Can you work these out from the model? Positions are in its coordinate system, mm. Face numbers are marked on the shaded views. Coordinates: 2 decimals unless noted, no trailing zeros. Loops run counter-clockwise (first coordinate to the right, second up) from the corner with the lowest first, then second, coordinate; pieces in that order, holes last. Notation, with made-up numbers: (-5.75, 26) -> (53.25, 26) arc R26 cw to (53.25, 47) -> close; hole circle Ø3 at (69.5, -1). An arc over 180 degrees is marked (long way). Put each result on its own line as item: value. Start each with the question number.
Item 1: If we section it at A-A on x = -34.75: Please give me the cut outline in (y, z).
Item 2: Will this pin go through, and if not, where does the flat tip stop? P1, Ø5, axis at y = -12.5, z = -5.5, coming from the -X side.
Item 3: If we section it at D-D on z = -4.5: Please give me the cut outline in (x, y), plus the area to 3 significant figures.
Item 4: If we section it at B-B on y = -17.5: Please give me the cut outline in (x, z), plus the area to 3 significant figures.
Item 5: We'd pull the mould along X, two halves only. Please class the marked faces 1, 2 and 3: pulls with the +X half, pulls with the -X half, needs draft (parallel to the pull), parting line crosses it, or undercut.
Item 6: Please list where these lines run through material, in increasing order: L1, parallel to X at y = -5.75, z = 0; L2, parallel to Z at x = -32, y = -3.75; L3, parallel to Z at x = -38, y = -3. Write a range as from..to.
Item 7: If we section it at C-C on z = 0: Please give me the cut outline in (x, y), plus the area to 3 significant figures.
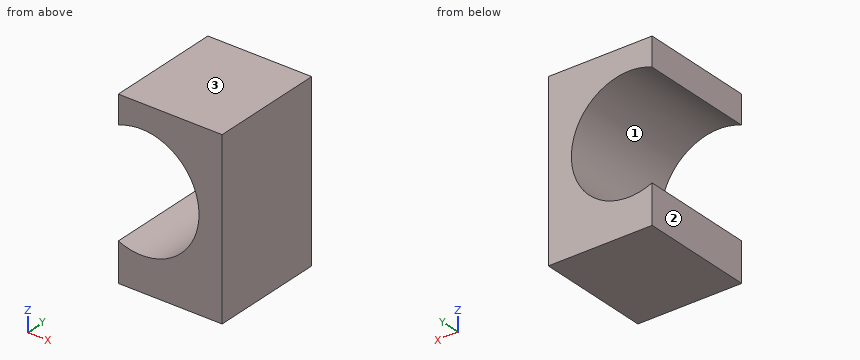
```python
from build123d import *

# Parameters (mm, degrees)
F0_W     = 22.86
F0_H     = 38.1
F1_DEPTH = 25.4
F2_R     = 12.7
F3_DEPTH = 89
F5_DEPTH = 25.401


# Not quite as in the source:
# - an extrude ends at something that could not be found from the text; its depth is read off the source's solid


with BuildPart() as f1:
    # F0 (on Front) → F1 (new body)
    with BuildSketch(Plane.XZ):
        with Locations((-34.8423583888, -1.1378988595)):
            Rectangle(F0_W, F0_H)
    extrude(amount=F1_DEPTH)

    # F2 (on Front) → F3 (cut, through all)
    with BuildSketch(Plane.XZ):
        with Locations((-35.3627614677, 3.7935657892)):
            Circle(F2_R)
    extrude(amount=-F3_DEPTH, mode=Mode.SUBTRACT)

    # F4 (on face) → F5 (cut, through all)
    with BuildSketch(Plane(origin=(0, 0, 0), x_dir=(-1, 0, 0), z_dir=(0, 1, 0))):
        with BuildLine():
            ThreePointArc((46.2723583888, -11.6417417865), (51.8211548639, -6.9581684388), (53.8969423294, 0))
            ThreePointArc((53.8969423294, 0), (51.8211548639, 6.9581684388), (46.2723583888, 11.6417417865))
            Line((46.2723583888, 11.6417417865), (46.2723583888, -11.6417417865))
        make_face()
        with BuildLine():
            Line((46.2723583888, -11.6417417865), (46.2723583888, 11.6417417865))
            ThreePointArc((46.2723583888, 11.6417417865), (28.4969423294, 0), (46.2723583888, -11.6417417865))
        make_face()
    extrude(amount=-F5_DEPTH, mode=Mode.SUBTRACT)


solid = f1.part
```
Solutions:
1. outline: (-25.4, -20.19) -> (0, -20.19) -> (0, -10.94) -> (-25.4, -10.94) -> close; (-25.4, 10.94) -> (0, 10.94) -> (0, 17.91) -> (-25.4, 17.91) -> close
2. P1: x = -31.33
3. outline: (-29.32, -25.4) -> (-23.41, -25.4) -> (-23.41, 0) -> (-29.32, 0) -> close
3. area: 150 mm^2
4. outline: (-46.27, -20.19) -> (-23.41, -20.19) -> (-23.41, 17.91) -> (-46.27, 17.91) -> (-46.27, 11.64) arc R12.7 cw (long way) to (-46.27, -11.64) -> close
4. area: 492 mm^2
5. face 1: undercut
5. face 2: pulls with the -X half
5. face 3: needs draft
6. L1: -28.5..-23.41
6. L2: -20.19..-8.76, 8.76..17.91
6. L3: -20.19..-12.29, 12.29..17.91
7. outline: (-28.5, -25.4) -> (-23.41, -25.4) -> (-23.41, 0) -> (-28.5, 0) -> close
7. area: 129 mm^2
